Geometry check sheet. Reference: the model listing, model coordinates, mm. A direction names the side the tool comes from. Coordinates: 2 decimals unless noted, no trailing zeros. Order: outer loops, then holes, each group sorted by start corner. A loop starts at its lowest first (then second) coordinate and runs counter-clockwise, first axis right, second up. Notation, with made-up numbers: M -10,64.25 L 37,64.25 A28 cw 37,89.25 Z; hole C 10,50.5 d3. An arc over 180 degrees is marked long. Use CSV: the item, a comma, the result in double quotes. Start each with the question number.
```python
from build123d import *


with BuildPart() as f2:
    # F2: sweep along a path in F1
    with BuildLine(Plane.YZ) as f2_path:
        Line((0, 5.226784), (83.332258, 5.226784))
        ThreePointArc((83.332258, 5.226784), (95.006591, 0.391117), (99.842258, -11.283216))
        Line((99.842258, -11.283216), (99.842258, -26.583992))
    # F0 (on Front) → F2 (sweep)
    with BuildSketch(Plane.XZ):
        Polygon((-1, -1.732051), (1, -1.732051), (2, 0), (1, 1.732051), (-1, 1.732051), (-2, 0), align=None)
    sweep(path=f2_path.line)


solid = f2.part
```
1) Section check C-C on y = 29. Record the boundary of the cut face in (x, z), then the cut area to 3 significant figures.
2) Gauge pin test, flat ends, axial feed: P1, Ø1.5, axis at x = 1, y = 72, coming from the -Z side; P2, Ø1, axis at x = 1, z = -8.5, coming from the +Y side; P3, Ø1.6, axis at x = 0, z = -22, coming from the -Y side. Record the tip position at first contact, or that the pin passes through.
3) Set-up check for faces 1 (the face through (0, 96.348, -19)), 2 (the face through (0, 92.883, -19)), 3 (the face through (1.493, 93.737, -19.041)), 4 (the face through (-1.507, 93.762, -19.041)), 5 (the face through (0, 95, -26.584)): record each of +Z, -Z, +X, -X, +Y, -Y from which the full face is reachable in a straight line by a thin tool's end or side.
4) Section check A-A on x = -0.05. Record the boundary of the cut face in (y, z).
5) Section check B-B on z = -19. Record the boundary of the cut face in (x, y).
6) Material ranges on line 1 along Z through (x, y) = (-0.25, 41); line 2 along Y through (x, z) = (0.45, -18); line 3 along X through (y, z) = (38.5, -1.5), recorded low to high.
Results are:
1,outline,"M -2,0 L -1,-1.73 L 1,-1.73 L 2,0 L 1,1.73 L -1,1.73 Z"
1,area,"10.4 mm²"
2,P1,"stops at z = -1.73"
2,P2,"stops at y = 96.15"
2,P3,"stops at y = 92.88"
3,face 1,"+Z, -Z, +X, -X, +Y"
3,face 2,"-Z, +X, -X, -Y"
3,face 3,"-Z, +X, -Y"
3,face 4,"-Z, -X, -Y"
3,face 5,"-Z, +X, -X, +Y, -Y"
4,outline,"M 0,-1.73 L 83.33,-1.73 A9.55 cw 92.88,-11.28 L 92.88,-26.58 L 96.35,-26.58 L 96.35,-11.28 A13.02 ccw 83.33,1.73 L 0,1.73 Z"
5,outline,"M -2,94.62 L -1,92.88 L 1,92.88 L 2,94.62 L 1,96.35 L -1,96.35 Z"
6,line 1,"z = -1.73 to 1.73"
6,line 2,"y = 92.88 to 96.35"
6,line 3,"x = -1.13 to 1.13"
